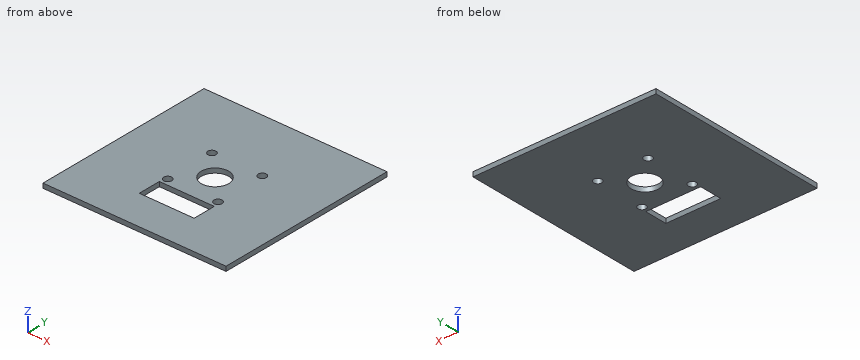
from build123d import *

# Parameters (mm, degrees)
SKETCH1_W           = 254
SKETCH1_H           = 254
SKETCH1_R           = 19.05
SKETCH1_R_2         = 5.603093475
SKETCH1_W_2         = 76.2
SKETCH1_H_2         = 31.75
BOSS_EXTRUDE1_DEPTH = 3.175


with BuildPart() as part:
    # Sketch1 → Boss-Extrude1 (new, symmetric)
    with BuildSketch(Plane.XY):
        Rectangle(SKETCH1_W, SKETCH1_H)
        Circle(SKETCH1_R, mode=Mode.SUBTRACT)
        with Locations((-34.925, 34.925)):
            Circle(SKETCH1_R_2, mode=Mode.SUBTRACT)
        with Locations((34.925, 34.925)):
            Circle(SKETCH1_R_2, mode=Mode.SUBTRACT)
        with Locations((-34.925, -34.925)):
            Circle(SKETCH1_R_2, mode=Mode.SUBTRACT)
        with Locations((34.925, -34.925)):
            Circle(SKETCH1_R_2, mode=Mode.SUBTRACT)
        with Locations((0, -60.325)):
            Rectangle(SKETCH1_W_2, SKETCH1_H_2, mode=Mode.SUBTRACT)
    extrude(amount=BOSS_EXTRUDE1_DEPTH, both=True)


solid = part.part
Input: part model. Units: mm. Frame: model coordinates. Round coordinates to 2 decimals unless told otherwise and drop trailing zeros. Loops run counter-clockwise (first coordinate to the right, second up) from the corner with the lowest first, then second, coordinate; pieces in that order, holes last. Notation, with made-up numbers: M 7.5,67 L 40.5,67 A4 ccw 40.5,74 Z; hole C -7.5,26.5 d6. An arc over 180 degrees is marked long. Answer as CSV lines item,"result". Start each with the question number.
(1) Section B-B, the plane x = 0. Output: boundary loops of the cut face in (y, z) (3 decimals).
(2) Line query: line 1 (Y direction, x = 0, z = -0.25); line 2 (Y direction, x = 30.5, z = 0.75); line 3 (Y direction, x = 2.5, z = -2). Output: solid intervals per line, ascending. Write a range as [from, to].
(3) Section A-A, the plane y = -50. Output: boundary loops of the cut face in (x, z) (3 decimals), plus the area to 3 significant figures.
(4) Section C-C, the plane z = 0.5. Output: boundary loops of the cut face in (x, y) (3 decimals).
(5) Section D-D, the plane y = 0. Output: boundary loops of the cut face in (x, z) (3 decimals), plus the area to 3 significant figures.
Values found:
1,outline,"M -127,-3.175 L -76.2,-3.175 L -76.2,3.175 L -127,3.175 Z; M -44.45,-3.175 L -19.05,-3.175 L -19.05,3.175 L -44.45,3.175 Z; M 19.05,-3.175 L 127,-3.175 L 127,3.175 L 19.05,3.175 Z"
2,line 1,"y = [-127, -76.2], [-44.45, -19.05], [19.05, 127]"
2,line 2,"y = [-127, -76.2], [-44.45, -38.36], [-31.49, 31.49], [38.36, 127]"
2,line 3,"y = [-127, -76.2], [-44.45, -18.89], [18.89, 127]"
3,outline,"M -127,-3.175 L -38.1,-3.175 L -38.1,3.175 L -127,3.175 Z; M 38.1,-3.175 L 127,-3.175 L 127,3.175 L 38.1,3.175 Z"
3,area,"1,130 mm²"
4,outline,"M -127,-127 L 127,-127 L 127,127 L -127,127 Z; hole C -34.925,-34.925 d11.206; hole C -34.925,34.925 d11.206; hole M -38.1,-76.2 L 38.1,-76.2 L 38.1,-44.45 L -38.1,-44.45 Z; hole C 0,0 d38.1; hole C 34.925,-34.925 d11.206; hole C 34.925,34.925 d11.206"
5,outline,"M -127,-3.175 L -19.05,-3.175 L -19.05,3.175 L -127,3.175 Z; M 19.05,-3.175 L 127,-3.175 L 127,3.175 L 19.05,3.175 Z"
5,area,"1,370 mm²"
